```python
from build123d import *

# Parameters (mm, degrees)
F0_W     = 4.5
F0_H     = 4.5
F1_DEPTH = 20
F3_DEPTH = 4


with BuildPart() as f1:
    # F0 (on Top) → F1 (new body)
    with BuildSketch(Plane.XY):
        with Locations((2.25, 2.25)):
            Rectangle(F0_W, F0_H)
    extrude(amount=F1_DEPTH)

    # F2 (on face) → F3 (join)
    with BuildSketch(Plane.XY.offset(20)):
        with BuildLine():
            Line((0.25, 2.25), (2.25, 2.25))
            Line((2.25, 2.25), (2.25, 4.25))
            ThreePointArc((2.25, 4.25), (0.8357864376, 3.6642135624), (0.25, 2.25))
        make_face()
        with BuildLine():
            Line((2.25, 2.25), (4.25, 2.25))
            ThreePointArc((4.25, 2.25), (3.6642135624, 3.6642135624), (2.25, 4.25))
            Line((2.25, 4.25), (2.25, 2.25))
        make_face()
        with BuildLine():
            ThreePointArc((2.25, 0.25), (3.6642135624, 0.8357864376), (4.25, 2.25))
            Line((4.25, 2.25), (2.25, 2.25))
            Line((2.25, 2.25), (2.25, 0.25))
        make_face()
        with BuildLine():
            Line((2.25, 0.25), (2.25, 2.25))
            Line((2.25, 2.25), (0.25, 2.25))
            ThreePointArc((0.25, 2.25), (0.8357864376, 0.8357864376), (2.25, 0.25))
        make_face()
    extrude(amount=F3_DEPTH)


solid = f1.part
```
Input: part model. Units: mm. Frame: model coordinates. Round coordinates to 2 decimals unless told otherwise and drop trailing zeros. Order: outer loops, then holes, each group sorted by start corner. A loop starts at its lowest first (then second) coordinate and runs counter-clockwise, first axis right, second up. Notation, with made-up numbers: (-12, -16.5) - (16, -16.5) arc R31 cw to (16, 12.5) - close; hole circle Ø2 at (69.5, -23.75). An arc over 180 degrees is marked (long way). One line per question, with ' | ' between items. Start each with the question number.
1) Cut plane B-B, the plane y = 3.6. Return the cut outline in (x, z).
2) Cut plane C-C, the plane z = 22.5. Return the cut outline in (x, y).
3) Cut plane A-A, the plane x = 3.85. Return the cut outline in (y, z), then the cut area to 3 significant figures.
4) Ray query, probe 1 along Z at (x, y) = (4.2, 4.05); probe 2 along X at (y, z) = (2.1, 21.5); probe 3 along Y at (x, z) = (1.45, 22.5). Return the intervals inside material, ascending.
Worked out:
1) outline: (0, 0) - (4.5, 0) - (4.5, 20) - (3.73, 20) - (3.73, 24) - (0.77, 24) - (0.77, 20) - (0, 20) - close
2) outline: circle Ø4 at (2.25, 2.25)
3) outline: (0, 0) - (4.5, 0) - (4.5, 20) - (3.45, 20) - (3.45, 24) - (1.05, 24) - (1.05, 20) - (0, 20) - close | area: 99.6 mm^2
4) probe 1: z = 0 to 20 | probe 2: x = 0.26 to 4.24 | probe 3: y = 0.42 to 4.08
